Autodesk Inventor part; units mm, degrees
ref_plane "YZ Plane" through (0, 0, 0) normal (1, 0, 0) x (0, 1, 0)
ref_plane "XZ Plane" through (0, 0, 0) normal (0, 1, 0) x (-1, 0, 0)
ref_plane "XY Plane" through (0, 0, 0) normal (0, 0, 1) x (1, 0, 0)
sketch "Esquisse1" plane through (0, 0, 0) normal (0, 1, 0) x (-1, 0, 0)
  line L0 (21.1354, -34.867) -> (21.1354, 40.133)
  circle A0 centre (1.447, -25.4161) radius 1.75
  circle A1 centre (1.447, -15.4161) radius 1.75
  circle A2 centre (8.3757, -15.4161) radius 1.75
  circle A3 centre (1.447, -4.8968) radius 1.75
  circle A4 centre (8.3757, -25.4161) radius 1.75
  line L1 (11.1354, 10.1032) -> (11.1354, -9.8968)
  line L2 (11.1354, -9.8968) -> (21.1354, -9.8968)
  line L3 (21.1354, -9.8968) -> (21.1354, 10.1032)
  line L4 (21.1354, 10.1032) -> (11.1354, -9.8968)
  line L5 (11.1354, 10.1032) -> (21.1354, -9.8968)
  line L6 (21.1354, 10.1032) -> (11.1354, 10.1032)
  line L7 (-18.8646, -34.867) -> (21.1354, -34.867)
  line L8 (-18.8646, -34.867) -> (21.1354, -34.867)
  line L9 (21.1354, -34.867) -> (21.1354, 40.133)
  line L10 (-18.8646, 40.133) -> (-18.8646, -34.867)
  line L11 (21.1354, 40.133) -> (-18.8646, 40.133)
  circle A5 centre (-68.4692, 33.6895) radius 1.75
  circle A6 centre (-68.4692, 42.6792) radius 1.75
  circle A7 centre (-4.9148, -25.4161) radius 1.75
  circle A8 centre (-4.9148, -15.4161) radius 1.75
  circle A9 centre (-4.9148, -4.8968) radius 1.75
  circle A10 centre (-12.188, -25.4161) radius 1.75
  circle A11 centre (-12.188, -15.4161) radius 1.75
  circle A12 centre (-12.188, -4.8968) radius 1.75
  circle A13 centre (15, -15.4161) radius 1.75
  circle A14 centre (15, -25.4161) radius 1.75
  circle A15 centre (1.447, 21.6987) radius 1.75
  circle A16 centre (1.447, 32.218) radius 1.75
  circle A17 centre (8.3757, 32.218) radius 1.75
  circle A18 centre (8.3757, 21.6987) radius 1.75
  circle A19 centre (-4.9148, 32.218) radius 1.75
  circle A20 centre (-4.9148, 21.6987) radius 1.75
  circle A21 centre (-12.188, 32.218) radius 1.75
  circle A22 centre (-12.188, 21.6987) radius 1.75
  circle A23 centre (15, 32.218) radius 1.75
  circle A24 centre (15, 21.6987) radius 1.75
  circle A25 centre (1.447, 10.1642) radius 1.75
  circle A26 centre (-4.9148, 10.1193) radius 1.75
  circle A27 centre (-12.188, 10.1193) radius 1.75
  point P0 (0, 0)
  point P1 (-36.8646, 0.1032)
  point P2 (-36.8646, 0.1032)
  point P3 (30.1354, 0.1032)
  point P4 (-36.8646, 0.1032)
  point P5 (16.1354, 0.1032)
  dimension "d28" = 40
  dimension "d30" = 75
extrude "Extrusion1" add sketch "Esquisse1" along normal blind 3 contours L7 L10 L11 L0 L6 L1 L2
sketch "Esquisse2" plane through (0, 0, 0) normal (0, -1, 0) x (1, 0, 0)
  line L0 (18.8646, -34.867) -> (-21.1354, -34.867)
  line L1 (-21.1354, -34.867) -> (-21.1354, -9.8968)
  line L2 (-7.3354, -28.867) -> (-17.3354, -28.867)
  line L3 (-17.3354, -28.867) -> (-17.3354, -31.867)
  line L4 (-17.3354, -31.867) -> (-7.3354, -31.867)
  line L5 (-7.3354, -31.867) -> (-7.3354, -28.867)
  line L6 (-7.3354, -28.867) -> (-17.3354, -31.867) construction
  line L7 (-17.3354, -28.867) -> (-7.3354, -31.867) construction
  line L8 (-21.1354, 10.1032) -> (-21.1354, 40.133)
  line L9 (-21.1354, 40.133) -> (18.8646, 40.133)
  line L10 (-17.3354, 34.133) -> (-7.3354, 34.133)
  line L11 (-7.3354, 34.133) -> (-7.3354, 37.133)
  line L12 (-7.3354, 37.133) -> (-17.3354, 37.133)
  line L13 (-17.3354, 37.133) -> (-17.3354, 34.133)
  line L14 (-17.3354, 34.133) -> (-7.3354, 37.133) construction
  line L15 (-7.3354, 34.133) -> (-17.3354, 37.133) construction
  point P0 (0, 0)
  point P1 (-12.3354, -30.367)
  point P2 (-12.3354, 35.633)
  point P3 (-17.3354, -34.867)
  point P4 (-7.3354, -34.867)
  point P5 (-7.3354, 40.133)
  point P6 (-17.3354, 40.133)
  dimension "d34" = 8.8
  dimension "d35" = 4.5
  dimension "d36" = 10
  dimension "d37" = 3
  dimension "d38" = 8.8
  dimension "d39" = 4.5
  dimension "d40" = 10
  dimension "d41" = 3
sketch "Esquisse4" plane through (-21.1354, 3, 40.133) normal (0, 0, 1) x (1, 0, 0)
  line L0 (10, -3) -> (0, -3)
  line L1 (13.8, -3) -> (13.8, -13)
  line L2 (3.7966, -3) -> (13.8, -13)
  line L3 (13.8, -13) -> (13.8, -3)
  line L4 (13.8, -3) -> (3.8, -13.0034)
  circle A0 centre (8.8, -8) radius 1.75
  circle A1 centre (8.8, -8) radius 1.75
  point P0 (21.1354, -3)
  dimension "d48" = 3.5
extrude "Extrusion5" cut sketch "Esquisse4" against normal blind 3 contours A0 L2 L4 | L4 L2 A0 | A0 L4 L2 | L4 A0 L2
extrude "Extrusion6" add sketch "Esquisse2" along normal blind 10
sketch "Esquisse5" plane through (-7.3354, 0, -31.867) normal (0, 0, -1) x (-1, 0, 0)
  line L0 (0, -10) -> (10, 0)
  line L1 (10, 0) -> (10, -10)
  line L2 (0, 0) -> (0, -10)
  line L3 (10, -10) -> (0, 0)
  circle A0 centre (5, -5) radius 1.75
  point P0 (-7.3354, 0)
  dimension "d56" = 3.5
extrude "Extrusion8" cut sketch "Esquisse5" against normal blind 3 contours A0 L3 L0 | L0 L3 A0 | L3 A0 L0 | L0 A0 L3
sketch "Esquisse6" plane through (-17.3354, 0, 37.133) normal (0, 0, 1) x (1, 0, 0)
  line L0 (10, -10) -> (0, 0)
  line L1 (6.2, 0) -> (-3.8, 0)
  line L2 (0, 0) -> (0, -10)
  line L3 (0, -10) -> (10, 0)
  line L4 (-3.8, 0) -> (36.2, 0)
  circle A0 centre (5, -5) radius 1.75
  point P0 (17.3354, 0)
  dimension "d61" = 3.5
extrude "Extrusion9" cut sketch "Esquisse6" against normal blind 3 contours A0 L3 L0 | L0 L3 A0 | L3 A0 L0 | L0 A0 L3
fillet "Congé3" radius 2 4 edges at (-17.3354, -10, 35.633) (-7.3354, -10, 35.633) (-17.3354, -10, -30.367) (-7.3354, -10, -30.367)
fillet "Congé4" radius 2 2 edges at (-17.3354, 0, -30.367) (-17.3354, 0, 35.633)
fillet "Congé5" radius 2 2 edges at (-7.3354, 0, -30.367) (-7.3354, 0, 35.633)
properties part number "étage_servo"
Work out the finished part from the listing and answer in its coordinate system (mm). A direction names the side the tool comes from. Coordinates: 2 decimals unless noted, no trailing zeros. Write each loop counter-clockwise with the first axis right and the second up, starting at its lowest first coordinate (ties: lowest second). Pieces come first, ordered by that corner, then holes. Notation, with made-up numbers: M -14.5,22 L 17.5,22 A18 cw 17.5,37 Z; hole C -26,-33 d4. An arc over 180 degrees is marked long. Use one line per item in the form item = value. Start each with the question number.
1. The part is cut by section A-A (y = -5). Give the vertices of the cut face in (x, z).
2. The part is cut by section D-D (z = -18.5). Give the vertices of the cut face in (x, y).
3. A tool of negligible diameter and unlimited length cuts with its end or side. For faces 5 (the face through (-7.335, -5, -30)), 6 (the face through (11.38, 1.48, 23.25)), 7 (the face through (-11.135, 1, 0)), from which of +Z, -Z, +X, -X, +Y, -Y can it reach the whole face along a straight path? Write none if from no direction.
4. The part is cut by section C-C (y = -8.75). Give the vertices of the cut face in (x, z).
5. Each of these flat-tipped pins is pushed along its axis until it touches: P1, Ø3.5, axis at y = -5.5, z = 35.5, coming from the -X side; P2, Ø3, axis at x = -8.38, z = -15.42, coming from the +Y side; P3, Ø8, axis at x = -1, z = -2.5, coming from the -Y side; P4, Ø0.9, axis at y = 1.5, z = 3.5, coming from the -X side. Where does it stop, or does it pass through?
6. Straight lines are drawn through the part: probe 1 along Z at (x, y) = (-15, 2.1); probe 2 along Z at (x, y) = (-13.5, -2.75); probe 3 along Z at (x, y) = (-13.5, 1.5). For each, find the intervals that lie inside material, in ascending order. Write a range as from..to.
7. The part is cut by section B-B (x = 11.5). Give the vertices of the cut face in (y, z), plus the area to 3 significant figures.
8. The mould has two halves that part along X. Classify faces 1 (the face through (-7.94, -9.43, -30.35)), 2 (the face through (-14, -4, 34.133)), 3 (the face through (10.52, 1.48, -15.94)), 4 (the face through (-9.18, 1.48, -23.86)): released by +X, released by -X, zero draft, split by the parting line, or undercut.
Evaluation:
q1.outline = M -17.34,-31.87 L -14.09,-31.87 L -14.09,-28.87 L -17.34,-28.87 Z; M -17.34,34.13 L -14.09,34.13 L -14.09,37.13 L -17.34,37.13 Z; M -10.59,-31.87 L -7.34,-31.87 L -7.34,-28.87 L -10.59,-28.87 Z; M -10.59,34.13 L -7.34,34.13 L -7.34,37.13 L -10.59,37.13 Z
q2.outline = M -21.14,0 L 18.86,0 L 18.86,3 L -21.14,3 Z
q3.face_5 = +Z, -Z, +X, -Y
q3.face_6 = +Y, -Y
q3.face_7 = -X, +Y, -Y
q4.outline = M -17.19,-31.87 L -7.48,-31.87 L -7.48,-28.87 L -17.19,-28.87 Z; M -17.19,34.13 L -7.48,34.13 L -7.48,37.13 L -17.19,37.13 Z
q5.P1 = -17.34
q5.P2 = through
q5.P3 = 0
q5.P4 = -11.14
q6.probe_1 = -34.87..-27.17, -23.67..-17.17, -13.67..-9.9, 10.1..19.95, 23.45..30.47, 33.97..40.13
q6.probe_2 = -31.87..-28.87, 34.13..37.13
q6.probe_3 = -34.87..-26.32, -24.51..-16.32, -14.51..-9.9, 10.1..20.8, 22.6..31.32, 33.12..40.13
q7.outline = M 0,-34.87 L 3,-34.87 L 3,-27.03 L 0,-27.03 Z; M 0,-23.81 L 3,-23.81 L 3,-17.03 L 0,-17.03 Z; M 0,-13.81 L 3,-13.81 L 3,-6.51 L 0,-6.51 Z; M 0,-3.29 L 3,-3.29 L 3,8.51 L 0,8.51 Z; M 0,11.73 L 3,11.73 L 3,20.09 L 0,20.09 Z; M 0,23.31 L 3,23.31 L 3,30.61 L 0,30.61 Z; M 0,33.83 L 3,33.83 L 3,40.13 L 0,40.13 Z
q7.area = 167 mm^2
q8.face_1 = released by +X
q8.face_2 = zero draft
q8.face_3 = undercut
q8.face_4 = undercut
